from build123d import *

# Parameters (mm, degrees)
BOSS_EXTRUDE1_DEPTH = 6


with BuildPart() as part:
    # Sketch2 → Boss-Extrude1 (new body)
    with BuildSketch(Plane(origin=(0, 0, 0), x_dir=(1, 0, 0), z_dir=(0, 1, 0))):
        Polygon((0, 270), (0, 240.585), (6, 240.585), (6, 216.195), (0, 216.195), (0, 191.805), (6, 191.805), (6, 167.415), (0, 167.415), (0, 143.025), (0, 138), (19.415, 138), (19.415, 144), (43.805, 144), (43.805, 138), (68.195, 138), (68.195, 144), (92.585, 144), (92.585, 138), (112, 138), (112, 167.415), (106, 167.415), (106, 191.805), (112, 191.805), (112, 216.195), (106, 216.195), (106, 240.585), (112, 240.585), (112, 264.975), (112, 270), (92.585, 270), (92.585, 264), (68.195, 264), (68.195, 270), (43.805, 270), (43.805, 264), (19.415, 264), (19.415, 270), align=None)
    extrude(amount=BOSS_EXTRUDE1_DEPTH)


solid = part.part
The listing builds one solid part. Answer for the finished solid, in the listing's coordinates (mm). A direction names the side the tool comes from. Give positions to 0.01 mm unless a question says otherwise; leave off trailing zeros. Loops run counter-clockwise (first coordinate to the right, second up) from the corner with the lowest first, then second, coordinate; pieces in that order, holes last. Notation, with made-up numbers: M 69,51 L 108,51 A23 cw 108,80 Z; hole C -32.75,44 d5. An arc over 180 degrees is marked long. Answer as CSV lines item,"result".
Item 1: Which of the six approach directions +Z, -Z, +X, -X, +Y, -Y give full straight-line access (tool end or side, diameter ignored) to faces 4 (the flat face through (3, 3, -240.585)), 5 (the flat face through (81, 3, -264)), 6 (the flat face through (19.415, 3, -141)), 7 (the flat face through (56, 3, -270)), 8 (the flat face through (106, 3, -228))?
Values follow:
face 4,"-X, +Y, -Y"
face 5,"-Z, +Y, -Y"
face 6,"+Z, +Y, -Y"
face 7,"-Z, +X, -X, +Y, -Y"
face 8,"+X, +Y, -Y"
Item 2: Given pin 1 Ø3 at (x, y) = (26.5, 2) entering from +Z; pin 2 Ø1.8 at (x, y) = (36.5, 3) entering from -Z, each flat-ended and moving along its own axis, determine where each tip first touches the part or whether it passes through.
Values follow:
pin 1,"stops at z = -144"
pin 2,"stops at z = -264"
Item 3: Straight lines are drawn through the part: line 1 along X through (y, z) = (1.8, -231.5); line 2 along Z through (x, y) = (82, 2.75). For each, find the intervals that lie inside material, in ascending order. Write a range as [from, to].
Values follow:
line 1,"x = [6, 106]"
line 2,"z = [-264, -144]"
Item 4: The part is cut by section B-B (z = -189). Give the vertices of the cut face in (x, y).
Values follow:
outline,"M 6,0 L 106,0 L 106,6 L 6,6 Z"
Item 5: The mould has two halves that part along Z. Classify faces 1 (the flat face through (43.805, 3, -267)), 2 (the flat face through (109, 3, -216.195)), 3 (the flat face through (10, 3, -138)): released by +Z, released by -Z, zero draft, split by the parting line, or undercut.
Values follow:
face 1,"zero draft"
face 2,"undercut"
face 3,"released by +Z"
Item 6: The part is cut by section A-A (x = 26). Give the vertices of the cut face in (y, z), and give its area (3 significant figures).
Values follow:
outline,"M 0,-264 L 6,-264 L 6,-144 L 0,-144 Z"
area,"720 mm^2"
